```python
from build123d import *

# Parameters (mm, degrees)
PAD_DEPTH    = 25
SKETCH001_R  = 48
PAD001_DEPTH = 48
SKETCH002_R  = 50
POCKET_DEPTH = 51


with BuildPart() as part:
    # Sketch → Pad (new body, symmetric)
    with BuildSketch(Plane.XY):
        with BuildLine():
            ThreePointArc((0, 125), (-125, 0), (0, -125))
            Line((0, -125), (500, -75))
            ThreePointArc((500, -75), (575, 0), (500, 75))
            Line((0, 125), (500, 75))
        make_face()
    extrude(amount=PAD_DEPTH, both=True)

    # Sketch001 (on Face5 of Pad) → Pad001 (join)
    with BuildSketch(Plane(origin=(0, 0, -25), x_dir=(1, 0, 0), z_dir=(0, 0, -1))):
        Circle(SKETCH001_R)
    extrude(amount=PAD001_DEPTH)

    # Sketch002 (on Face5 of Pad001) → Pocket (cut)
    with BuildSketch(Plane.XY.offset(25)):
        with Locations((500, 0)):
            Circle(SKETCH002_R)
    extrude(amount=-POCKET_DEPTH, mode=Mode.SUBTRACT)


solid = part.part
```
Part model, mm, in its own coordinate system. A direction names the side the tool comes from. Give positions to 0.01 mm unless a question says otherwise; leave off trailing zeros. Loops run counter-clockwise (first coordinate to the right, second up) from the corner with the lowest first, then second, coordinate; pieces in that order, holes last. Notation, with made-up numbers: M 80,26 L 120,26 A34 ccw 120,61 Z; hole C 71,-1 d9. An arc over 180 degrees is marked long. Return JSON: item names as keys, results as strings.
1) Saw through at D-D, the plane y = 106. List the corners of the cut face in (x, z).
Calculated:
{"outline": "M -66.25,-25 L 190,-25 L 190,25 L -66.25,25 Z"}
2) 3-axis set-ups, long thin cutter, end or side, ignore diameter. For faces 1 (the face through (-47.954, -2.11, -48.664)), 2 (the face through (-124.97, 2.75, 0.35)): which of +Z, -Z, +X, -X, +Y, -Y reach the whole face in a straight line?
Calculated:
{"face 1": "-Z", "face 2": "+Z, -Z, -X"}
3) Drill centre lines: line 1 (Y direction, x = 500, z = -13); line 2 (Z direction, x = 77.5, y = 66); line 3 (Y direction, x = 466.5, z = -6.5). Where is each one in solid material? Low to high.
Calculated:
{"line 1": "y = -75 to -50, 50 to 75", "line 2": "z = -25 to 25", "line 3": "y = -78.35 to -37.12, 37.12 to 78.35"}
4) Flat gauge pins, fed straight in: pin 1 Ø2 at (x, z) = (412.5, -5) entering from +Y; pin 2 Ø12 at (x, z) = (278, 11) entering from +Y; pin 3 Ø4 at (x, z) = (294.5, -9) entering from -Y. Where does each tip first touch, or does it go through?
Calculated:
{"pin 1": "stops at y = 83.85", "pin 2": "stops at y = 97.8", "pin 3": "stops at y = -95.75"}
5) Pull direction X, two halves, no side cores. Call faces 3 (the face through (246.5, -100.35, 0.35)), 4 (the face through (-1, -1, -73)), 5 (the face through (547.69, 15.02, 0.35)): released by +X, released by -X, zero draft, split by the parting line, or undercut.
Calculated:
{"face 3": "released by +X", "face 4": "zero draft", "face 5": "undercut"}
6) Saw through at A-A, the plane y = 0. List the corners of the cut face in (x, z), then the cut area to 3 significant figures.
Calculated:
{"outline": "M -125,-25 L -48,-25 L -48,-73 L 48,-73 L 48,-25 L 450,-25 L 450,25 L -125,25 Z; M 550,-25 L 575,-25 L 575,25 L 550,25 Z", "area": "34,600 mm2"}
7) Saw through at B-B, the plane z = -13.5. List the corners of the cut face in (x, y).
Calculated:
{"outline": "M 0,-125 L 500,-75 A75 ccw 500,75 L 0,125 A125 ccw Z; hole C 500,0 d100"}
8) Saw through at C-C, the plane x = 270. List the corners of the cut face in (y, z), then the cut area to 3 significant figures.
Calculated:
{"outline": "M -98,-25 L 98,-25 L 98,25 L -98,25 Z", "area": "9,800 mm2"}
